The listing builds one solid part. Answer for the finished solid, in the listing's coordinates (mm). Face numbers are marked on the shaded views. Round coordinates to 2 decimals unless told otherwise and drop trailing zeros. Loops run counter-clockwise (first coordinate to the right, second up) from the corner with the lowest first, then second, coordinate; pieces in that order, holes last. Notation, with made-up numbers: (88.5, -36.5) -> (126.5, -36.5) arc R35 cw to (126.5, 2.5) -> close; hole circle Ø11 at (-27, 87.5). An arc over 180 degrees is marked (long way). Use a Markdown table: item, result. Add a question column.
Q1. For a pull along Z with two mould halves and no side action, classify the marked faces 1 and 2 as released by +Z, released by -Z, zero draft, split by the parting line, or undercut.
Q2. Section D-D on y = -19.9 is taken. Give the vertices of the cut face in (x, z).
Q3. Given pin 1 Ø1.5 at (x, y) = (-50, -12.5) entering from -Z; pin 2 Ø1.5 at (x, z) = (-37.5, 64.5) entering from -Y; pin 3 Ø8 at (x, z) = (-91, 7.5) entering from +Y; pin 4 Ø3 at (x, y) = (-49, -25) entering from -Z, each flat-ended and moving along its own axis, determine where each tip first touches the part or whether it passes through.
Q4. Consider line 1 (Z direction, x = -9, y = -2); line 2 (X direction, y = -2, z = 7); line 3 (Z direction, x = -22, y = -19.9). Determine where each line is inside the solid, lowest interval first.
Q5. Section A-A on z = 7.5 is taken. Give the vertices of the cut face in (x, y), then the cut area to 3 significant figures.
Q6. Section B-B on x = -91 is taken. Give the vertices of the cut face in (y, z).
Q7. Section C-C on y = -1.5 is taken. Give the vertices of the cut face in (x, z), then the cut area to 3 significant figures.
from build123d import *

# Parameters (mm, degrees)
F0_W     = 100
F0_H     = 77
F1_DEPTH = 5
F3_D     = 10
F4_R     = 12
F5_DEPTH = 100


with BuildPart() as f1:
    # F0 (on Front) → F1 (new body)
    with BuildSketch(Plane.XZ):
        with Locations((-50, 38.5)):
            Rectangle(F0_W, F0_H)
    extrude(amount=F1_DEPTH)

    # F3 (through all)
    with Locations(Plane.XZ.offset(5)):
        with Locations((-91, 69.5), (-9, 69.5), (-91, 7.5), (-9, 7.5)):
            Hole(F3_D / 2)

    # F4 (on face) → F5 (join, through all)
    with BuildSketch(Plane(origin=(-100, 0, 0), x_dir=(0, -1, 0), z_dir=(-1, 0, 0))):
        with BuildLine():
            ThreePointArc((5, 36.770838), (20.766025, 23.525021), (34.9, 38.5))
            ThreePointArc((34.9, 38.5), (20.766025, 53.474979), (5, 40.229162))
            Line((5, 40.229162), (5, 36.770838))
        make_face()
        with Locations((19.9, 38.5)):
            Circle(F4_R, mode=Mode.SUBTRACT)
    extrude(amount=-F5_DEPTH)


solid = f1.part
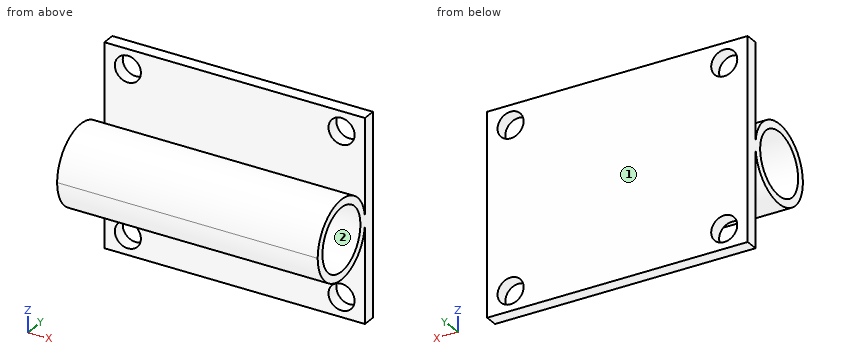
Checked values:
| question | item | result |
|---|---|---|
| 1 | face 1 | zero draft |
| 1 | face 2 | undercut |
| 2 | outline | (-100, 23.5) -> (0, 23.5) -> (0, 26.5) -> (-100, 26.5) -> close; (-100, 50.5) -> (0, 50.5) -> (0, 53.5) -> (-100, 53.5) -> close |
| 3 | pin 1 | stops at z = 25.05 |
| 3 | pin 2 | stops at y = -5 |
| 3 | pin 3 | passes through |
| 3 | pin 4 | stops at z = 23.94 |
| 4 | line 1 | z = 0 to 2.5, 12.5 to 64.5, 74.5 to 77 |
| 4 | line 2 | x = -100 to -95.97, -86.03 to -13.97, -4.03 to 0 |
| 4 | line 3 | z = 23.5 to 26.5, 50.5 to 53.5 |
| 5 | outline | (-100, -5) -> (-96, -5) -> (-96, 0) -> (-100, 0) -> close; (-86, -5) -> (-14, -5) -> (-14, 0) -> (-86, 0) -> close; (-4, -5) -> (0, -5) -> (0, 0) -> (-4, 0) -> close |
| 5 | area | 400 mm2 |
| 6 | outline | (-5, 0) -> (0, 0) -> (0, 2.5) -> (-5, 2.5) -> close; (-5, 12.5) -> (0, 12.5) -> (0, 64.5) -> (-5, 64.5) -> (-5, 40.23) arc R15 ccw (long way) to (-5, 36.77) -> close; (-5, 74.5) -> (0, 74.5) -> (0, 77) -> (-5, 77) -> close; hole circle Ø24 at (-19.9, 38.5) |
| 7 | outline | (-100, 0) -> (0, 0) -> (0, 77) -> (-100, 77) -> close; hole circle Ø10 at (-91, 7.5); hole circle Ø10 at (-91, 69.5); hole circle Ø10 at (-9, 7.5); hole circle Ø10 at (-9, 69.5) |
| 7 | area | 7,390 mm2 |
